Autodesk Inventor part; units mm, degrees
ref_plane "YZ Plane" through (0, 0, 0) normal (1, 0, 0) x (0, 1, 0)
ref_plane "XZ Plane" through (0, 0, 0) normal (0, 1, 0) x (-1, 0, 0)
ref_plane "XY Plane" through (0, 0, 0) normal (0, 0, 1) x (1, 0, 0)
sketch "Sketch1" plane through (0, 0, 0) normal (0, 1, 0) x (-1, 0, 0)
  circle A0 centre (0, 0) radius 10.75
  dimension "d0" = 21.5
extrude "Extrusion1" add sketch "Sketch1" along normal blind 11
sketch "Sketch2" plane through (0, 11, 0) normal (0, 1, 0) x (1, 0, 0)
  circle A0 centre (0, 0) radius 10
  dimension "d3" = 20
extrude "Extrusion2" cut sketch "Sketch2" against normal blind 10
fillet "Fillet1" radius 1.5 1 edges at (10.75, 0, 0)
fillet "Fillet2" radius 0.25 2 edges at (10.75, 11, 0) (-10, 11, 0)
thread "Thread1"
sketch "Sketch3" plane through (0, 1, 0) normal (0, 1, 0) x (1, 0, 0)
  point P0 (0, 0)
sketch "Sketch4" plane through (0, 0, 0) normal (0, -1, 0) x (1, 0, 0)
  line L0 (-6.0026, 1.747) -> (5.8016, 1.747) construction
  line L1 (5.8016, 1.747) -> (5.8016, -1.301) construction
  line L2 (5.8016, -1.301) -> (-6.0026, -1.301) construction
  line L3 (-6.0026, -1.301) -> (-6.0026, 1.747) construction
  point P0 (0, 0)
properties part number "kork 32"
CAD build for the part. Positions are in the model's coordinates, mm. Coordinates: 2 decimals unless noted, no trailing zeros. Order: outer loops, then holes, each group sorted by start corner. A loop starts at its lowest first (then second) coordinate and runs counter-clockwise, first axis right, second up. Notation, with made-up numbers: (-8, 42) - (30, 42) arc R12 cw to (30, 47) - close; hole circle Ø3 at (65.25, 53.25). An arc over 180 degrees is marked (long way). Use a Markdown table: item, result. Add a question column.
(1) Saw through at A-A (x = 0). Give the cut face in (y, z), then the cut area to 3 significant figures.
(2) Drill centre lines: line 1 along Z through (x, y) = (0, 8.5); line 2 along Y through (x, z) = (5.5, 6.25); line 3 along Z through (x, y) = (-4.75, 2.25). Where is each one in solid material? Low to high. Write a range as [from, to].
(3) Saw through at B-B (z = 0). Give the cut face in (x, y), then the cut area to 3 significant figures.
(4) Saw through at C-C (y = 2.75). Give the cut face in (x, z).
(5) Pull direction Z, two halves, no side cores. Call faces 1 (the face through (-2.17, 5.94, 9.76)), 2 (the face through (0, 0, 0)), 3 (the face through (1.4, 6.06, -10.66)): +Z half, -Z half, draft (parallel to the pull), parting line (faces both ways), or undercut.
(6) Flat gauge pins, fed straight in: pin 1 (2 mm diameter, centred on x = 1.5, y = 8, fed in from +Z); pin 2 (1 mm diameter, centred on y = 4, z = 1.5, fed in from -X); pin 3 (10 mm diameter, centred on x = 3, z = -2, fed in from +Y). Where does each tip first touch, or does it go through?
Solved:
| question | item | result |
|---|---|---|
| 1 | outline | (0, -9.25) arc R1.5 ccw to (1.5, -10.75) - (10.75, -10.75) arc R0.25 ccw to (11, -10.5) - (11, -10.25) arc R0.25 ccw to (10.75, -10) - (1, -10) - (1, 10) - (10.75, 10) arc R0.25 ccw to (11, 10.25) - (11, 10.5) arc R0.25 ccw to (10.75, 10.75) - (1.5, 10.75) arc R1.5 ccw to (0, 9.25) - close |
| 1 | area | 35.5 mm² |
| 2 | line 1 | z = [-10.75, -10], [10, 10.75] |
| 2 | line 2 | y = [0, 1] |
| 2 | line 3 | z = [-9.64, -8.8], [8.8, 9.64] |
| 3 | outline | (-10.75, 1.5) arc R1.5 ccw to (-9.25, 0) - (9.25, 0) arc R1.5 ccw to (10.75, 1.5) - (10.75, 10.75) arc R0.25 ccw to (10.5, 11) - (10.25, 11) arc R0.25 ccw to (10, 10.75) - (10, 1) - (-10, 1) - (-10, 10.75) arc R0.25 ccw to (-10.25, 11) - (-10.5, 11) arc R0.25 ccw to (-10.75, 10.75) - close |
| 3 | area | 35.5 mm² |
| 4 | outline | circle Ø21.5 at (0, 0); hole circle Ø20 at (0, 0) |
| 5 | face 1 | undercut |
| 5 | face 2 | draft |
| 5 | face 3 | parting line |
| 6 | pin 1 | stops at z = 10.74 |
| 6 | pin 2 | stops at x = -10.7 |
| 6 | pin 3 | stops at y = 1 |
